Design review of the part built by this model. Coordinates are the model's own, in mm. Face numbers are marked on the shaded views. A direction names the side the tool comes from. Give positions to 0.01 mm unless a question says otherwise; leave off trailing zeros. Order: outer loops, then holes, each group sorted by start corner. A loop starts at its lowest first (then second) coordinate and runs counter-clockwise, first axis right, second up. Notation, with made-up numbers: (8, 61.25) -> (43, 61.25) arc R22 cw to (43, 78.25) -> close; hole circle Ø3 at (64.25, 5.25). An arc over 180 degrees is marked (long way). One line per item, written item: value.
from build123d import *
from build123d.topology import SkipClean

# Parameters (mm, degrees)
BASEFRAMESKETCH_W    = 15.38
BASEFRAMESKETCH_H    = 3.2
BASEFRAME_DEPTH      = 7.9
SKETCH29_W           = 15.38
SKETCH29_H           = 7.9
CUT_EXTRUDE4_DEPTH   = 16.116827041
SKETCH31_R           = 2.197938665
BOSS_EXTRUDE6_DEPTH  = 1.6
LPATTERN4_COUNT      = 2
LPATTERN4_PITCH      = 8
SHELL1_T             = -1.2
BOSS_EXTRUDE7_DEPTH  = 2.3
CUT_EXTRUDE7_DEPTH   = 2.3
FILLET3_R            = 0.1
FILLET4_R            = 0.1
SKETCH38_W           = 7.69
SKETCH38_H           = 7.9
CUT_EXTRUDE8_DEPTH   = 4
BOSS_EXTRUDE16_START = 0.8
SKETCH44_R           = 0.997938665
BOSS_EXTRUDE16_DEPTH = 0.8
BOSS_EXTRUDE17_REACH = 13.769
SKETCH39_W           = 1.2
SKETCH39_H           = 5.5
CUT_EXTRUDE10_DEPTH  = 12.768845427
SKETCH46_W           = 0.335
SKETCH46_H           = 3.2
SKETCH100_W          = 0.349019596
SKETCH100_H          = 5.5
SKETCH101_W          = 0.3
SKETCH101_H          = 5.5
CUT_EXTRUDE27_DEPTH  = 11.500279785
SKETCH104_W          = 1.97
SKETCH104_H          = 1.97
CUT_EXTRUDE28_DEPTH  = 1.6
SWEEP27_START        = 2
SWEEP27_DEPTH        = 0.4
MOVE_FACE1_BY        = 3.3
CUT_EXTRUDE42_DEPTH  = 14.215613325
SKETCH118_R          = 2.4
SKETCH118_R_2        = 1.8
BOSS_EXTRUDE26_DEPTH = 1.6
SKETCH119_R          = 1.8
CUT_EXTRUDE43_DEPTH  = 12.160161573
SKETCH120_W          = 7.69000258
SKETCH120_H          = 3.3
CUT_EXTRUDE44_DEPTH  = 11.263488994
SKETCH121_R          = 1.8
BOSS_EXTRUDE27_DEPTH = 2.8


# Read off the part's stored shape, not the designer's step: Sweep27
with BuildPart() as part:
    # BaseFrameSketch → BaseFrame (new, symmetric)
    with BuildSketch(Plane.XY):
        with Locations((-4.794729064, 1.6)):
            Rectangle(BASEFRAMESKETCH_W, BASEFRAMESKETCH_H)
    extrude(amount=BASEFRAME_DEPTH, both=True)

    # Sketch29 → Cut-Extrude4 (cut, through all)
    with BuildSketch(Plane(origin=(0, 3.2, 0), x_dir=(1, 0, 0), z_dir=(0, 1, 0))):
        with Locations((-4.794729064, 3.95)):
            Rectangle(SKETCH29_W, SKETCH29_H)
    extrude(amount=-CUT_EXTRUDE4_DEPTH, mode=Mode.SUBTRACT)

    # Sketch31 → Boss-Extrude6 (add)
    with BuildSketch(Plane(origin=(0, 3.2, 0), x_dir=(1, 0, 0), z_dir=(0, 1, 0))):
        with Locations((-8.584729064, -4)):
            Circle(SKETCH31_R)
    boss_extrude6 = extrude(amount=BOSS_EXTRUDE6_DEPTH)

    # LPattern4: Boss-Extrude6 ×2
    with Locations(*[(i * LPATTERN4_PITCH, 0, 0) for i in range(1, LPATTERN4_COUNT)]):
        add(boss_extrude6)

    # Shell1
    shell1_openings = [part.faces().sort_by_distance(p)[0] for p in [
        (-4.794729064, 0, 3.95),
    ]]
    offset(amount=SHELL1_T, openings=shell1_openings, kind=Kind.INTERSECTION)

    # Sketch35 → Boss-Extrude7 (add, symmetric)
    with BuildSketch(Plane.XY.offset(3.95)):
        with BuildLine():
            Line((-2.782667729, 3.2), (1.613209601, 3.2))
            ThreePointArc((1.613209601, 3.2), (1.721005084, 3.313571782), (1.810586387, 3.441999215))
            ThreePointArc((1.810586387, 3.441999215), (2.278525574, 4.313545175), (2.440270936, 5.289453921))
            ThreePointArc((2.440270936, 5.289453921), (2.428474077, 6.289536316), (2.360954202, 7.287406564))
            Line((2.360954202, 7.287406564), (1.106266226, 7.287406564))
            ThreePointArc((1.106266226, 7.287406564), (1.22292125, 6.096651625), (1.106266226, 4.905896686))
            ThreePointArc((1.106266226, 4.905896686), (-0.584729064, 4.033269084), (-2.275724354, 4.905896686))
            ThreePointArc((-2.275724354, 4.905896686), (-2.392379378, 6.096651625), (-2.275724354, 7.287406564))
            Line((-2.275724354, 7.287406564), (-3.53041233, 7.287406564))
            ThreePointArc((-3.53041233, 7.287406564), (-3.597932205, 6.289536316), (-3.609729064, 5.289453921))
            ThreePointArc((-3.609729064, 5.289453921), (-3.447983702, 4.313545175), (-2.980044515, 3.441999215))
            ThreePointArc((-2.980044515, 3.441999215), (-2.890463212, 3.313571782), (-2.782667729, 3.2))
        make_face()
    extrude(amount=BOSS_EXTRUDE7_DEPTH, both=True)

    # Sketch36 → Cut-Extrude7 (cut, symmetric)
    with BuildSketch(Plane.XY.offset(3.95)):
        with BuildLine():
            Line((-2.195211087, 4.8), (1.025752959, 4.8))
            ThreePointArc((1.025752959, 4.8), (-0.584729064, 4.033269084), (-2.195211087, 4.8))
        make_face()
    extrude(amount=CUT_EXTRUDE7_DEPTH, both=True, mode=Mode.SUBTRACT)

    # Fillet3
    fillet3_edges = [part.edges().sort_by_distance(p)[0] for p in [
        (-2.275724354, 4.905896686, 3.95),
    ]]
    fillet(fillet3_edges, radius=FILLET3_R)

    # Fillet4
    fillet4_edges = [part.edges().sort_by_distance(p)[0] for p in [
        (1.106266226, 4.905896686, 3.95),
    ]]
    fillet(fillet4_edges, radius=FILLET4_R)

    # Sketch38 → Cut-Extrude8 (cut, symmetric)
    with BuildSketch(Plane(origin=(0, 3.2, 0), x_dir=(1, 0, 0), z_dir=(0, 1, 0))):
        with Locations((-8.639729064, -3.95)):
            Rectangle(SKETCH38_W, SKETCH38_H)
    extrude(amount=CUT_EXTRUDE8_DEPTH, both=True, mode=Mode.SUBTRACT)

    # Sketch44 → Boss-Extrude16 (add)
    with BuildSketch(Plane.XZ.offset(-3.2).offset(BOSS_EXTRUDE16_START)):
        with Locations((-0.584729064, 4)):
            Circle(SKETCH44_R)
    extrude(amount=-BOSS_EXTRUDE16_DEPTH)

    # Sketch39 → Boss-Extrude17 (add, up to next)
    with BuildSketch(Plane(origin=(0, 0, 0), x_dir=(-1, 0, 0), z_dir=(0, -1, 0)), mode=Mode.PRIVATE) as boss_extrude17_sk1:
        with Locations((4.194729064, -3.95)):
            Rectangle(SKETCH39_W, SKETCH39_H)
    boss_extrude17_tool1 = extrude(boss_extrude17_sk1.sketch, amount=-BOSS_EXTRUDE17_REACH, mode=Mode.PRIVATE) - part.part
    add(boss_extrude17_tool1.solids().sort_by_distance((-4.194729, 0, 3.95))[0])

    # Sketch45 → Cut-Extrude10 (cut, through all)
    with BuildSketch(Plane.XY.offset(7.9)):
        Polygon((-4.794729064, 3.2), (-4.459731644, 3.2), (-4.459731644, 0), (-4.794729064, -0.001314844), align=None)
    extrude(amount=-CUT_EXTRUDE10_DEPTH, mode=Mode.SUBTRACT)

    # Sweep9: sweep along a curve in space
    with BuildLine() as sweep9_path:
        Line((2.895270936, 3.2, 7.9), (2.895270936, 3.2, 0))
    # Sketch46 → Sweep9 (sweep)
    with BuildSketch(Plane.XY.offset(7.9)):
        with Locations((3.062770936, 1.6)):
            Rectangle(SKETCH46_W, SKETCH46_H)
    sweep(path=sweep9_path.line)

    # Sweep24: sweep along a curve in space
    with BuildLine() as sweep24_path:
        Line((-3.594729064, 2, 6.7), (-3.594729064, 0, 6.7))
    # Sketch100 → Sweep24 (sweep)
    with BuildSketch(Plane(origin=(0, 2, 0), x_dir=(-1, 0, 0), z_dir=(0, -1, 0))):
        with Locations((3.420219266, -3.95)):
            Rectangle(SKETCH100_W, SKETCH100_H)
    sweep(path=sweep24_path.line)

    # Sketch101 → Cut-Extrude27 (cut, through all)
    with BuildSketch(Plane(origin=(0, 2, 0), x_dir=(-1, 0, 0), z_dir=(0, -1, 0))):
        with Locations((-1.845270936, -3.95)):
            Rectangle(SKETCH101_W, SKETCH101_H)
    extrude(amount=CUT_EXTRUDE27_DEPTH, mode=Mode.SUBTRACT)

    # Sketch104 → Cut-Extrude28 (cut)
    with BuildSketch(Plane(origin=(0, 2, 0), x_dir=(-1, 0, 0), z_dir=(0, -1, 0))):
        with Locations((0.625219266, -3.95)):
            Rectangle(SKETCH104_W, SKETCH104_H)
    extrude(amount=-CUT_EXTRUDE28_DEPTH, mode=Mode.SUBTRACT)

    # Sweep27 outline → Sweep27 (add)
    with BuildSketch(Plane(origin=(0, 0, 0), x_dir=(1, 0, 0), z_dir=(0, 1, 0)).offset(SWEEP27_START)):
        with BuildLine():
            Line((0.359780734, -3.677846589), (0.359780734, -4.322153411))
            ThreePointArc((0.359780734, -4.322153411), (0.413209601, -4), (0.359780734, -3.677846589))
        make_face()
        with BuildLine():
            Line((-0.235936032, -4.935), (-0.933522096, -4.935))
            ThreePointArc((-0.933522096, -4.935), (-0.584729064, -4.997938665), (-0.235936032, -4.935))
        make_face()
    extrude(amount=SWEEP27_DEPTH)

    # Move Face1: a face moved outward by 3.3
    extrude(part.faces().sort_by_distance((-0.614730354, 0, 0.79))[0], amount=MOVE_FACE1_BY, dir=(0, -1, 0))

    # Sketch115 → Cut-Extrude42 (cut, through all)
    with BuildSketch(Plane.ZY.offset(4.459731644)):
        Polygon((0, 3.2), (7.9, 3.2), (7.9, 7.494096257), (-0.222033581, 7.422914641), (-0.222033581, 3.2), align=None)
    extrude(amount=-CUT_EXTRUDE42_DEPTH, mode=Mode.SUBTRACT)

    # Sketch118 → Boss-Extrude26 (add)
    with BuildSketch(Plane(origin=(0, 3.2, 0), x_dir=(1, 0, 0), z_dir=(0, 1, 0))):
        with Locations((-0.614730354, -3.95)):
            Circle(SKETCH118_R)
        with Locations(Location((-0.614730354, -3.95, 0), (0, 0, 180))):
            Circle(SKETCH118_R_2, mode=Mode.SUBTRACT)
    extrude(amount=BOSS_EXTRUDE26_DEPTH)

    # Sketch119 → Cut-Extrude43 (cut, through all)
    with SkipClean():  # the faces are left unmerged after this step: merging them gives an invalid solid
        with BuildSketch(Plane(origin=(0, 3.2, 0), x_dir=(1, 0, 0), z_dir=(0, 1, 0))):
            with Locations((-0.614730354, -3.95)):
                Circle(SKETCH119_R)
        extrude(amount=-CUT_EXTRUDE43_DEPTH, mode=Mode.SUBTRACT)

    # Sketch120 → Cut-Extrude44 (cut, through all)
    with SkipClean():  # the faces are left unmerged after this step: merging them gives an invalid solid
        with BuildSketch(Plane.XY.offset(7.9)):
            with Locations((-0.614730354, -1.65)):
                Rectangle(SKETCH120_W, SKETCH120_H)
        extrude(amount=-CUT_EXTRUDE44_DEPTH, mode=Mode.SUBTRACT)

    # Sketch121 → Boss-Extrude27 (add)
    with BuildSketch(Plane(origin=(0, 2, 0), x_dir=(-1, 0, 0), z_dir=(0, -1, 0))):
        with Locations((0.614730354, -3.95)):
            Circle(SKETCH121_R)
    extrude(amount=-BOSS_EXTRUDE27_DEPTH)


solid = part.part
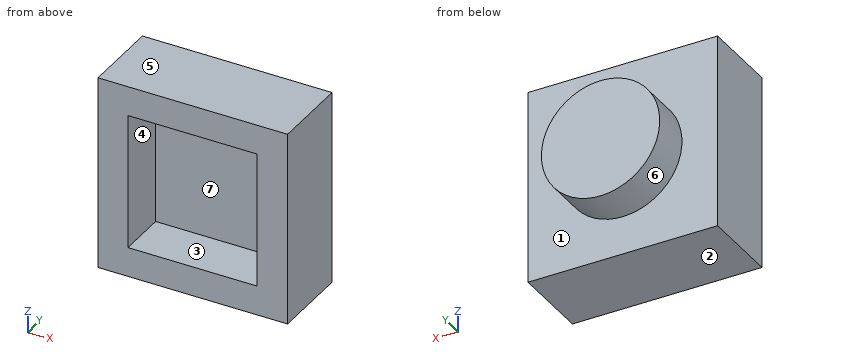
Item 1: To check wall thickness, follow line 1 along X through (y, z) = (0.7, 2); line 2 along Y through (x, z) = (1, 4.5); line 3 along Y through (x, z) = (1.75, 2.75). State the ranges of each line that lie inside material, in increasing order. Write a range as from..to.
Returned:
line 1: -4.46..-3.25, 2..3.23
line 2: 2..4.8
line 3: 2..3.2
Item 2: Clearance check with a flat-ended pin moving along its axis: P1, Ø1.6, axis at x = 0.5, z = 4.5, coming from the -Y side. State where the tip first meets the part, or that it passes through.
Returned:
P1: y = 2
Item 3: Machinability: for the marked faces 1, 2 and 3, which of the approach directions +Z, -Z, +X, -X, +Y, -Y give a long, thin tool a straight path to every point of the face, cutting with its end or side? Answer none if there is none.
Returned:
face 1: +Y
face 2: -Z, +X, -X, +Y, -Y
face 3: -Y
Item 4: Add section A-A on y = 1.5. Give the boundary of the cut face in (x, z).
Returned:
outline: (-4.46, 0) -> (3.23, 0) -> (3.23, 7.9) -> (-4.46, 7.9) -> close; hole (-3.25, 1.2) -> (2, 1.2) -> (2, 6.7) -> (-3.25, 6.7) -> close
Item 5: Add section D-D on y = 4. Give the boundary of the cut face in (x, z), plus the area to 3 significant figures.
Returned:
outline: circle Ø4.8 at (-0.61, 3.95)
area: 18.1 mm²
Item 6: Add section B-B on z = 3.95. Give the boundary of the cut face in (x, y).
Returned:
outline: (-4.46, 0) -> (-3.25, 0) -> (-3.25, 2) -> (2, 2) -> (2, 0) -> (3.23, 0) -> (3.23, 3.2) -> (1.79, 3.2) -> (1.79, 4.8) -> (-3.01, 4.8) -> (-3.01, 3.2) -> (-4.46, 3.2) -> close
Item 7: Draft analysis for pull direction Z (two halves, no side actions). For the marked faces 4, 5, 6 and 7, state which applies: pulls with the +Z half, pulls with the -Z half, needs draft (parallel to the pull), parting line crosses it, or undercut.
Returned:
face 4: undercut
face 5: pulls with the +Z half
face 6: parting line crosses it
face 7: undercut
Item 8: Add section C-C on x = -1.5. Give the boundary of the cut face in (y, z), plus the area to 3 significant figures.
Returned:
outline: (0, 0) -> (3.2, 0) -> (3.2, 1.72) -> (4.8, 1.72) -> (4.8, 6.18) -> (3.2, 6.18) -> (3.2, 7.9) -> (0, 7.9) -> (0, 6.7) -> (2, 6.7) -> (2, 1.2) -> (0, 1.2) -> close
area: 21.4 mm²
